Job drawing, mm, ordinate dimensions from the low corner. One solid piece. A direction names the side the tool comes from. Give positions to 0.01 mm unless a question says otherwise; leave off trailing zeros. Loops run counter-clockwise (first coordinate to the right, second up) from the corner with the lowest first, then second, coordinate; pieces in that order, holes last. Notation, with made-up numbers: M -28.75,67 L 24.25,67 A16 ccw 24.25,82 Z; hole C -23.5,54.5 d9. An arc over 180 degrees is marked long. One line per question, with ' | ' between items.
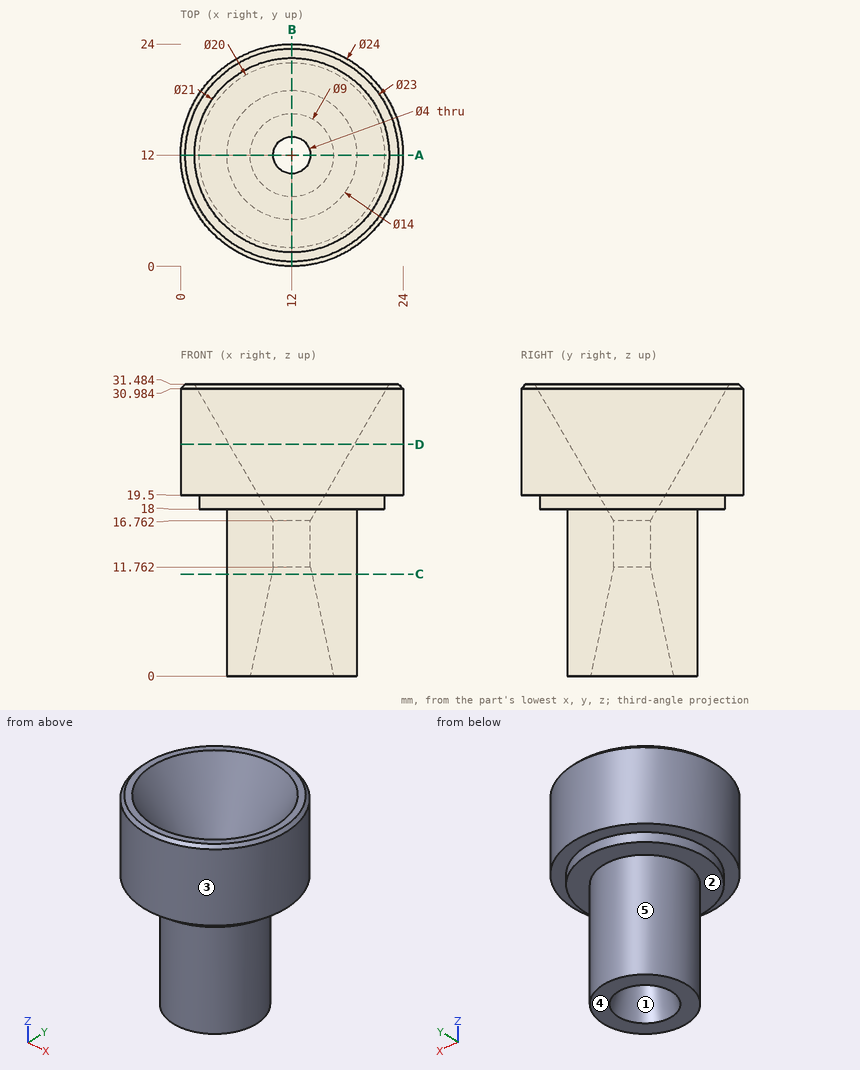
Item 1: Drop flat-ended pins along their axis: P1, Ø8, axis at x = 6.5, z = 3.5, coming from the +Y side; P2, Ø1.5, axis at x = 13, z = 9, coming from the +Y side; P3, Ø6, axis at x = 6.5, z = 22.5, coming from the -Y side. Give the stop position or say it passes through.
Conclusion:
P1: y = 18.84 | P2: y = 19 | P3: y = 0.26
Item 2: Saw through at C-C on z = 11. Give the cut face in (x, y).
Conclusion:
outline: C 12,12 d14; hole C 12,12 d4.32
Item 3: Saw through at D-D on z = 25. Give the cut face in (x, y).
Conclusion:
outline: C 12,12 d24; hole C 12,12 d13.51
Item 4: Saw through at A-A on y = 12. Give the cut face in (x, z).
Conclusion:
outline: M 0,19.5 L 2,19.5 L 2,18 L 5,18 L 5,0 L 7.5,0 L 10,11.76 L 10,16.76 L 1.5,31.48 L 0.5,31.48 L 0,30.98 Z; M 14,11.76 L 16.5,0 L 19,0 L 19,18 L 22,18 L 22,19.5 L 24,19.5 L 24,30.98 L 23.5,31.48 L 22.5,31.48 L 14,16.76 Z
Item 5: Mould opens along Y. For the marked faces 1, 2 and 3 say: pulls with the +Y half, pulls with the -Y half, needs draft (parallel to the pull), parting line crosses it, or undercut.
Conclusion:
face 1: undercut | face 2: needs draft | face 3: parting line crosses it
Item 6: 3-axis set-ups, long thin cutter, end or side, ignore diameter. For the marked faces 4 and 5: which of +Z, -Z, +X, -X, +Y, -Y reach the whole face in a straight line?
Conclusion:
face 4: -Z, +X, -X, +Y, -Y | face 5: -Z
Item 7: Drill centre lines: line 1 along X through (y, z) = (12, 14.6); line 2 along Y through (x, z) = (17, 23) (1 decimal); line 3 along Y through (x, z) = (9, 20.5). Where is each one in solid material? Low to high. Write a range as [from, to].
Conclusion:
line 1: [5, 10], [14, 19] | line 2: [1.1, 9.5], [14.5, 22.9] | line 3: [0.38, 9.12], [14.88, 23.62]
